from build123d import *

# Parameters (mm, degrees)
SKETCH2_W               = 100
SKETCH2_H               = 70
BOSS_EXTRUDE1_DEPTH     = 150
CUT_EXTRUDE1_DEPTH      = 184.643676722
CUT_EXTRUDE2_DEPTH      = 162.941347407
CUT_EXTRUDE2_DEPTH_BACK = 162.941347407
SHELL1_T                = -3


with BuildPart() as part:
    # Sketch2 → Boss-Extrude1 (new body)
    with BuildSketch(Plane(origin=(0, 0, 0), x_dir=(1, 0, 0), z_dir=(0, 1, 0))):
        Rectangle(SKETCH2_W, SKETCH2_H)
    extrude(amount=BOSS_EXTRUDE1_DEPTH)

    # Sketch3 → Cut-Extrude1 (cut, through all)
    with BuildSketch(Plane.ZY.offset(50)):
        Polygon((-35, 20), (-19.2, 150), (-35, 150), align=None)
        Polygon((19.2, 150), (35, 20), (35, 150), align=None)
    extrude(amount=-CUT_EXTRUDE1_DEPTH, mode=Mode.SUBTRACT)

    # Sketch4 → Cut-Extrude2 (cut, two sides: drawn at the far end of the back side and taken through both)
    with BuildSketch(Plane.XY.offset(-CUT_EXTRUDE2_DEPTH_BACK)):
        Polygon((-50, 20), (-9.808333333, 150), (-50, 150), align=None)
        Polygon((50, 20), (9.808333333, 150), (50, 150), align=None)
    extrude(amount=CUT_EXTRUDE2_DEPTH + CUT_EXTRUDE2_DEPTH_BACK, mode=Mode.SUBTRACT)

    # Shell1
    shell1_openings = [part.faces().sort_by_distance(p)[0] for p in [
        (0, 150, 0),
        (0, 0, 0),
    ]]
    offset(amount=SHELL1_T, openings=shell1_openings, kind=Kind.INTERSECTION)


solid = part.part
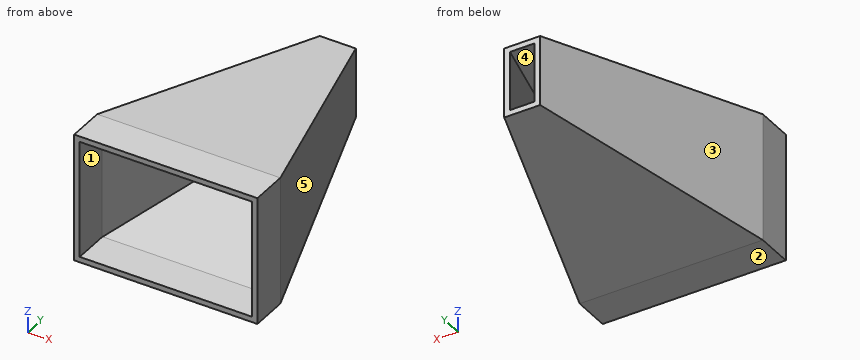
Design review of the part built by this model. Coordinates are the model's own, in mm. Face numbers are marked on the shaded views. A direction names the side the tool comes from. Round coordinates to 2 decimals unless told otherwise and drop trailing zeros. Loops run counter-clockwise (first coordinate to the right, second up) from the corner with the lowest first, then second, coordinate; pieces in that order, holes last. Notation, with made-up numbers: (52, -24.5) - (96, -24.5) arc R23 ccw to (96, -4.5) - close; hole circle Ø8 at (34.25, 41.5). An arc over 180 degrees is marked (long way). One line per item, written item: value. Start each with the question number.
1) Draft analysis for pull direction X (two halves, no side actions). For the marked faces 3, 4 and 5, state which applies: +X half, -X half, draft (parallel to the pull), parting line (faces both ways), or undercut.
2) For the marked faces 1 and 2, list the 3-axis set-ups (+Z, -Z, +X, -X, +Y, -Y) from which the entire face can be reached by the end or side of a thin tool; tool diameter is ignored.
3) Insertion check: pin 1 Ø12 at (y, z) = (92, 18) entering from -X (3 decimals); pin 2 Ø10 at (x, y) = (-19, 120.5) entering from -Z; pin 3 Ø10 at (x, y) = (-38, 79.5) entering from -Z; pin 4 Ø12 at (x, y) = (-22, 79.5) entering from +Z. Each pin has a flat end and moves straight along its axis. Give the tip position at first contact, or say it passes through.
4) Consider section B-B on y = 13. Give the boundary of the cut face in (x, z), then the cut area to 3 significant figures.
5) Consider section A-A on x = 4.5. Give the boundary of the cut face in (y, z).
6) To check wall thickness, follow L1, parallel to Z at x = 34, y = 8; L2, parallel to X at y = 19, z = 28; L3, parallel to X at y = 86.5, z = 10.5. State the ranges of each line that lie inside material, in increasing order. Write a range as from..to.
7) Consider section C-C on z = -4. Give the boundary of the cut face in (x, y).
8) Consider section D-D on z = 25.5. Give the boundary of the cut face in (x, y), then the cut area to 3 significant figures.
Reported:
1. face 3: -X half
1. face 4: undercut
1. face 5: +X half
2. face 1: -Y
2. face 2: -Z, +X, -X, +Y, -Y
3. pin 1: stops at x = -29.595
3. pin 2: stops at z = -23.39
3. pin 3: passes through
3. pin 4: stops at z = 28.5
4. outline: (-50, -35) - (50, -35) - (50, 35) - (-50, 35) - close; hole (-47, -32) - (47, -32) - (47, 32) - (-47, 32) - close
4. area: 984 mm^2
5. outline: (0, -35) - (20, -35) - (150, -19.2) - (150, -16.18) - (19.82, -32) - (0, -32) - close; (0, 32) - (19.82, 32) - (150, 16.18) - (150, 19.2) - (20, 35) - (0, 35) - close
6. L1: z = -35..-32, 32..35
6. L2: x = -50..-47, 47..50
6. L3: x = -29.44..-26.3, 26.3..29.44
7. outline: (-50, 0) - (-47, 0) - (-47, 19.55) - (-6.67, 150) - (-9.81, 150) - (-50, 20) - close; (6.67, 150) - (47, 19.55) - (47, 0) - (50, 0) - (50, 20) - (9.81, 150) - close
8. outline: (-50, 0) - (-47, 0) - (-47, 19.55) - (-30.38, 73.3) - (30.38, 73.3) - (47, 19.55) - (47, 0) - (50, 0) - (50, 20) - (25.83, 98.16) - (-25.83, 98.16) - (-50, 20) - close
8. area: 1,930 mm^2
